Geometry: final body of the model. Coordinates: model frame, mm. Round coordinates to 2 decimals unless told otherwise and drop trailing zeros. Write each loop counter-clockwise with the first axis right and the second up, starting at its lowest first coordinate (ties: lowest second). Pieces come first, ordered by that corner, then holes. Notation, with made-up numbers: (25, 2.5) -> (84, 2.5) arc R35 ccw to (84, 37.5) -> close; hole circle Ø5 at (-25, -30). An arc over 180 degrees is marked (long way). Use one line per item in the form item = value. Start each with the question number.
1. Cut plane B-B, the plane z = -66. Return the cut outline in (x, y).
2. Cut plane C-C, the plane y = 191.5. Return the cut outline in (x, z).
3. Cut plane A-A, the plane x = 3.35. Return the cut outline in (y, z), plus the area to 3 significant figures.
4. Line query: L1, parallel to Y at x = 2.2, z = -370; L2, parallel to Y at x = 4.75, z = -30; L3, parallel to Y at x = 4.8, z = -47.5. Output: solid intervals per line, ascending.
```python
from build123d import *

# Parameters (mm, degrees)
SKETCH1_R           = 2.5
BOSS_EXTRUDE1_DEPTH = 6


with BuildPart() as part:
    # Sketch1 → Boss-Extrude1 (new body)
    with BuildSketch(Plane(origin=(0, 0, 0), x_dir=(0, 0, -1), z_dir=(1, 0, 0))):
        Polygon((0, 0), (400, 0), (400, 400), (200, 400), (0, 60), align=None)
        with Locations((30, 42)):
            Circle(SKETCH1_R, mode=Mode.SUBTRACT)
        with Locations(Location((30, 18, 0), (0, 0, 180))):
            Circle(SKETCH1_R, mode=Mode.SUBTRACT)
        with Locations((370, 18)):
            Circle(SKETCH1_R, mode=Mode.SUBTRACT)
        with Locations(Location((370, 42, 0), (0, 0, 180))):
            Circle(SKETCH1_R, mode=Mode.SUBTRACT)
    extrude(amount=BOSS_EXTRUDE1_DEPTH)


solid = part.part
```
Outcome:
q1.outline = (0, 0) -> (6, 0) -> (6, 172.2) -> (0, 172.2) -> close
q2.outline = (0, -400) -> (6, -400) -> (6, -77.35) -> (0, -77.35) -> close
q3.outline = (0, -400) -> (400, -400) -> (400, -200) -> (60, 0) -> (0, 0) -> close; hole circle Ø5 at (18, -370); hole circle Ø5 at (18, -30); hole circle Ø5 at (42, -370); hole circle Ø5 at (42, -30)
q3.area = 126,000 mm^2
q4.L1 = 0 to 15.5, 20.5 to 39.5, 44.5 to 400
q4.L2 = 0 to 15.5, 20.5 to 39.5, 44.5 to 111
q4.L3 = 0 to 140.75
